Work out the finished part from the listing and answer in its coordinate system (mm). Give positions to 0.01 mm unless a question says otherwise; leave off trailing zeros. Loops run counter-clockwise (first coordinate to the right, second up) from the corner with the lowest first, then second, coordinate; pieces in that order, holes last. Notation, with made-up numbers: (75, 34) - (124, 34) arc R16 ccw to (124, 43) - close; hole circle Ø5 at (38.25, 31.25). An arc over 180 degrees is marked (long way). Use CSV: the item, a comma, the result in double quotes.
from build123d import *

# Parameters (mm, degrees)
SKETCH1_W           = 10
SKETCH1_H           = 20
BOSS_EXTRUDE1_DEPTH = 10
SKETCH3_R           = 1.5
CUT_EXTRUDE1_DEPTH  = 21
SKETCH2_R           = 1.5
BOSS_EXTRUDE2_DEPTH = 21


with BuildPart() as part:
    # Sketch1 → Boss-Extrude1 (new body)
    with BuildSketch(Plane(origin=(0, 0, 0), x_dir=(1, 0, 0), z_dir=(0, 1, 0))):
        with Locations((0.028248588, -7.485875706)):
            Rectangle(SKETCH1_W, SKETCH1_H)
    extrude(amount=BOSS_EXTRUDE1_DEPTH)

    # Sketch3 → Cut-Extrude1 (cut)
    with BuildSketch(Plane(origin=(0, 0, -2.514124294), x_dir=(-1, 0, 0), z_dir=(0, 0, -1))):
        with Locations((-0.028248588, 5)):
            Circle(SKETCH3_R)
    extrude(amount=-CUT_EXTRUDE1_DEPTH, mode=Mode.SUBTRACT)

    # Sketch2 → Boss-Extrude2 (add)
    with BuildSketch(Plane(origin=(0, 10, 0), x_dir=(1, 0, 0), z_dir=(0, 1, 0))):
        with Locations((0.028248588, -11.485875706)):
            Circle(SKETCH2_R)
    extrude(amount=BOSS_EXTRUDE2_DEPTH)


solid = part.part
Item 1: A cutting plane is placed at C-C on x = 0.25. Determine the outline of the cut face in (y, z), and give its area (3 significant figures).
Determined:
outline,"(0, -2.51) - (3.52, -2.51) - (3.52, 17.49) - (0, 17.49) - close; (6.48, -2.51) - (10, -2.51) - (10, 10) - (31, 10) - (31, 12.97) - (10, 12.97) - (10, 17.49) - (6.48, 17.49) - close"
area,"203 mm²"
Item 2: Given P1, Ø1.5, axis at y = 18, z = 14, coming from the +X side; P2, Ø1.5, axis at x = 0, y = 21, coming from the +Z side; P3, Ø6, axis at x = -1, z = 5.5, coming from the +Y side, each flat-ended and moving along its own axis, determine where each tip first touches the part or whether it passes through.
Determined:
P1,"passes through"
P2,"stops at z = 12.99"
P3,"stops at y = 10"
Item 3: Find the intervals of material crossed by line 1 (Y direction, x = 0, z = 1); line 2 (Y direction, x = 2.25, z = 14); line 3 (X direction, y = 4, z = 5), in increasing order.
Determined:
line 1,"y = 0 to 3.5, 6.5 to 10"
line 2,"y = 0 to 10"
line 3,"x = -4.97 to -1.09, 1.15 to 5.03"
Item 4: A cutting plane is placed at D-D on x = -4. Determine the outline of the cut face in (y, z).
Determined:
outline,"(0, -2.51) - (10, -2.51) - (10, 17.49) - (0, 17.49) - close"
Item 5: The mould has two halves that part along X. Classify faces 1 (the cylindrical face through (-1.402, 5.451, 7.346)), 2 (the flat face through (5.028, 5, 8)), 3 (the cylindrical face through (-0.3, 20.35, 12.95)), 4 (the flat face through (0, 0, 7)): pulls with the +X half, pulls with the -X half, needs draft (parallel to the pull), parting line crosses it, or undercut.
Determined:
face 1,"undercut"
face 2,"pulls with the +X half"
face 3,"parting line crosses it"
face 4,"needs draft"
Item 6: A cutting plane is placed at B-B on z = 3.25. Determine the outline of the cut face in (x, y), and give its area (3 significant figures).
Determined:
outline,"(-4.97, 0) - (5.03, 0) - (5.03, 10) - (-4.97, 10) - close; hole circle Ø3 at (0.03, 5)"
area,"92.9 mm²"
Item 7: A cutting plane is placed at A-A on y = 5. Determine the outline of the cut face in (x, z).
Determined:
outline,"(-4.97, -2.51) - (-1.47, -2.51) - (-1.47, 17.49) - (-4.97, 17.49) - close; (1.53, -2.51) - (5.03, -2.51) - (5.03, 17.49) - (1.53, 17.49) - close"
